```python
from build123d import *

# Parameters (mm, degrees)
SKETCH1_W                         = 120
SKETCH1_H                         = 50
BOSS_EXTRUDE1_DEPTH               = 10
SKETCH2_R                         = 1.5
LINEAR_BEARING_MOUNT_DEPTH        = 11
SKETCH3_R                         = 2.5
SURFACE_PROFILE_MOUNT_DEPTH       = 11
SKETCH4_R                         = 4.25
SURF_PROF_MOUNT_COUNTERSINK_DEPTH = 5
SKETCH5_R                         = 3.5
CUT_EXTRUDE1_DEPTH                = 4


with BuildPart() as part:
    # Sketch1 → Boss-Extrude1 (new body)
    with BuildSketch(Plane(origin=(0, 0, 0), x_dir=(1, 0, 0), z_dir=(0, 1, 0))):
        Rectangle(SKETCH1_W, SKETCH1_H)
    extrude(amount=BOSS_EXTRUDE1_DEPTH)

    # Sketch2 → Linear_bearing_mount (cut, through all)
    with BuildSketch(Plane(origin=(0, 10, 0), x_dir=(1, 0, 0), z_dir=(0, 1, 0))):
        with Locations((-28, -12)):
            Circle(SKETCH2_R)
        with Locations((-46, -12)):
            Circle(SKETCH2_R)
        with Locations((28, -12)):
            Circle(SKETCH2_R)
        with Locations((46, -12)):
            Circle(SKETCH2_R)
        with Locations((46, 12)):
            Circle(SKETCH2_R)
        with Locations((28, 12)):
            Circle(SKETCH2_R)
        with Locations((-46, 12)):
            Circle(SKETCH2_R)
        with Locations((-28, 12)):
            Circle(SKETCH2_R)
    extrude(amount=-LINEAR_BEARING_MOUNT_DEPTH, mode=Mode.SUBTRACT)

    # Sketch3 → Surface_profile_mount (cut, through all)
    with BuildSketch(Plane.XZ):
        Circle(SKETCH3_R)
        with Locations((30, 0)):
            Circle(SKETCH3_R)
        with Locations((-30, 0)):
            Circle(SKETCH3_R)
    extrude(amount=-SURFACE_PROFILE_MOUNT_DEPTH, mode=Mode.SUBTRACT)

    # Sketch4 → Surf.prof.mount_countersink (cut)
    with BuildSketch(Plane.XZ):
        with Locations((30, 0)):
            Circle(SKETCH4_R)
        Circle(SKETCH4_R)
        with Locations((-30, 0)):
            Circle(SKETCH4_R)
    extrude(amount=-SURF_PROF_MOUNT_COUNTERSINK_DEPTH, mode=Mode.SUBTRACT)

    # Sketch5 → Cut-Extrude1 (cut)
    with BuildSketch(Plane(origin=(0, 10, 0), x_dir=(1, 0, 0), z_dir=(0, 1, 0))):
        with Locations((-46, 12)):
            Circle(SKETCH5_R)
        with Locations((-28, 12)):
            Circle(SKETCH5_R)
        with Locations((-28, -12)):
            Circle(SKETCH5_R)
        with Locations((-46, -12)):
            Circle(SKETCH5_R)
        with Locations((46, -12)):
            Circle(SKETCH5_R)
        with Locations((28, -12)):
            Circle(SKETCH5_R)
        with Locations((28, 12)):
            Circle(SKETCH5_R)
        with Locations((46, 12)):
            Circle(SKETCH5_R)
    extrude(amount=-CUT_EXTRUDE1_DEPTH, mode=Mode.SUBTRACT)


solid = part.part
```
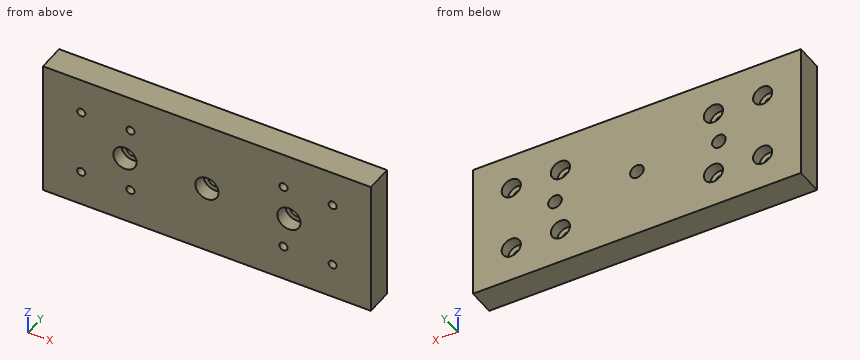
CAD build for the part. Positions are in the model's coordinates, mm. Round coordinates to 2 decimals unless told otherwise and drop trailing zeros. Order: outer loops, then holes, each group sorted by start corner. A loop starts at its lowest first (then second) coordinate and runs counter-clockwise, first axis right, second up. Notation, with made-up numbers: (51, 56) -> (98, 56) arc R5 ccw to (98, 63) -> close; hole circle Ø2 at (70.25, -35.75). An arc over 180 degrees is marked (long way). Write item = value, one per line.
(1) Cut at B-B (y = 3.25). State how many separate pieces and enclosed holes the cut face has, plus the area to 3 significant figures.
Answers follow:
separate_pieces = 1
enclosed_holes = 11
area = 5,770 mm²
(2) Cut at A-A (x = 46). Write the cut outline in (y, z), plus the area to 3 significant figures.
Answers follow:
outline = (0, -25) -> (10, -25) -> (10, -15.5) -> (6, -15.5) -> (6, -13.5) -> (0, -13.5) -> close; (0, -10.5) -> (6, -10.5) -> (6, -8.5) -> (10, -8.5) -> (10, 8.5) -> (6, 8.5) -> (6, 10.5) -> (0, 10.5) -> close; (0, 13.5) -> (6, 13.5) -> (6, 15.5) -> (10, 15.5) -> (10, 25) -> (0, 25) -> close
area = 408 mm²
(3) Flat gauge pins, fed straight in: P1, Ø2.5, axis at x = 28, z = -12, coming from the +Y side; P2, Ø4, axis at x = -29.5, z = 1, coming from the -Y side; P3, Ø6.5, axis at x = -28, z = 12, coming from the +Y side. Where does each tip first touch, or does it go through?
Answers follow:
P1 = through
P2 = 5
P3 = 6
(4) Cut at D-D (x = 0). Write the cut outline in (y, z), plus the area to 4 significant figures.
Answers follow:
outline = (0, -25) -> (10, -25) -> (10, -2.5) -> (5, -2.5) -> (5, -4.25) -> (0, -4.25) -> close; (0, 4.25) -> (5, 4.25) -> (5, 2.5) -> (10, 2.5) -> (10, 25) -> (0, 25) -> close
area = 432.5 mm²
(5) Drill centre lines: L1, parallel to X at y = 3.5, z = -12; L2, parallel to Z at x = -46, y = 3.75; L3, parallel to X at y = 8.4, z = -12. Where is each one in solid material? Low to high.
Answers follow:
L1 = -60 to -47.5, -44.5 to -29.5, -26.5 to 26.5, 29.5 to 44.5, 47.5 to 60
L2 = -25 to -13.5, -10.5 to 10.5, 13.5 to 25
L3 = -60 to -49.5, -42.5 to -31.5, -24.5 to 24.5, 31.5 to 42.5, 49.5 to 60
(6) Cut at C-C (z = 0). Write the cut outline in (x, y).
Answers follow:
outline = (-60, 0) -> (-34.25, 0) -> (-34.25, 5) -> (-32.5, 5) -> (-32.5, 10) -> (-60, 10) -> close; (-27.5, 5) -> (-25.75, 5) -> (-25.75, 0) -> (-4.25, 0) -> (-4.25, 5) -> (-2.5, 5) -> (-2.5, 10) -> (-27.5, 10) -> close; (2.5, 5) -> (4.25, 5) -> (4.25, 0) -> (25.75, 0) -> (25.75, 5) -> (27.5, 5) -> (27.5, 10) -> (2.5, 10) -> close; (32.5, 5) -> (34.25, 5) -> (34.25, 0) -> (60, 0) -> (60, 10) -> (32.5, 10) -> close
